Geometry check sheet. Reference: the model listing, model coordinates, mm. Face numbers are marked on the shaded views. A direction names the side the tool comes from. Give positions to 0.01 mm unless a question says otherwise; leave off trailing zeros. Loops run counter-clockwise (first coordinate to the right, second up) from the corner with the lowest first, then second, coordinate; pieces in that order, holes last. Notation, with made-up numbers: (-24.5, 86) -> (0.5, 86) arc R28 ccw to (0.5, 117) -> close; hole circle Ø9 at (52.5, 28). An arc over 180 degrees is marked (long way). One line per item, written item: value. Start each with the question number.
(1) Sectioned sample at C-C, the plane x = 18. Record the cut outline in (y, z), then the cut area to 3 significant figures.
(2) Gauge pin test, flat ends, axial feed: pin 1 Ø2.5 at (x, y) = (20.5, 1) entering from +Z; pin 2 Ø1 at (y, z) = (-1.5, 1) entering from -X; pin 3 Ø1.6 at (y, z) = (2, 43.5) entering from +X. Record the tip position at first contact, or that the pin passes through.
(3) Sectioned sample at B-B, the plane z = 24. Record the cut outline in (x, y).
(4) Tool access check on the marked faces 5 and 6. Record the directions out of +Z, -Z, +X, -X, +Y, -Y that give a thin tool (end or side, any length) a straight path to the whole face; none if there is none.
(5) Draft check along X on the marked faces 1, 2, 3 and 4. Enter one of: pulls with the +X half, pulls with the -X half, needs draft (parallel to the pull), parting line crosses it, or undercut.
(6) Scan lines: line 1 along X through (y, z) = (0, 25); line 2 along X through (y, z) = (1.75, 35.5); line 3 along Y through (x, z) = (40, 22). Record each from-to range of solid material in increasing order. Write a range as from..to.
(7) Sectioned sample at A-A, the plane y = 0. State how many separate pieces and enclosed holes the cut face has, then the cut area to 3 significant figures.
Autodesk Fusion 360 part; units mm, degrees
sketch "Sketch1" plane through (0, 0, 0) normal (0, 0, 1) x (1, 0, 0)
  circle A0 centre (0, 0) radius 2.65
  circle A1 centre (0, 0) radius 5
  line L0 (0, 0) -> (40, 0) construction
  circle A2 centre (40, 0) radius 2.65
  circle A3 centre (40, 0) radius 5
  line L1 (0, -5) -> (40, -5)
  line L2 (0, 5) -> (40, 5)
  dimension "d3" = 5.3
  dimension "d4" = 10
  dimension "d5" = 40
  dimension "d6" = 5.3
  dimension "d7" = 10
extrude "Extrude1" add sketch "Sketch1" along normal blind 45
chamfer "Chamfer1" distance 1 angle 45 2 edges at (-2.4707, 0.9583, 45) (37.5293, 0.9583, 45)
fillet "Fillet1" radius 2.5 2 edges at (-2.4707, 0.9583, 44) (37.5293, 0.9583, 44)
ref_plane "WorkPlane1" through (0, 0, 0) normal (1, 0, 0) x (0, 1, 0)
chamfer "Chamfer2" distance 1 angle 45 2 edges at (-2.4707, 0.9583, 0) (37.5293, 0.9583, 0)
sketch "Sketch2" plane through (0, -5, 0) normal (0, -1, 0) x (1, 0, 0)
  line L0 (0, 0) -> (40, 0)
  line L1 (40, 0) -> (40, 45)
  line L2 (40, 45) -> (0, 45)
  line L3 (0, 45) -> (0, 0)
  line L4 (20, 45) -> (20, 43)
  line L5 (20, 43) -> (16, 43)
  line L6 (16, 43) -> (16, 45)
  line L7 (16, 45) -> (20, 45)
  line L8 (20, 45) -> (20, 43)
  line L9 (20, 45) -> (24, 45)
  line L10 (24, 45) -> (24, 43)
  line L11 (24, 43) -> (20, 43)
  line L12 (20, 43) -> (20, 45)
  line L13 (20, 0) -> (16, 0)
  line L14 (16, 0) -> (16, 2)
  line L15 (16, 2) -> (20, 2)
  line L16 (20, 2) -> (20, 0)
  line L17 (20, 0) -> (24, 0)
  line L18 (24, 0) -> (24, 2)
  line L19 (24, 2) -> (20, 2)
  line L20 (20, 2) -> (20, 0)
  dimension "d15" = 2
  dimension "d16" = 4
  dimension "d17" = 4
  dimension "d18" = 4
  dimension "d19" = 2
  dimension "d20" = 4
  dimension "d21" = 2
extrude "Extrude2" cut sketch "Sketch2" against normal blind 14 contours L0 L13 L14 L15 L16 L20 | L0 L16 L17 L18 L19 L20 | L2 L4 L5 L6 L7 L8 L12 | L2 L4 L8 L9 L10 L11 L12
fillet "Fillet2" radius 2.5 2 edges at (-2.4707, -0.9583, 1) (37.5293, -0.9583, 1)
equation "spacing = 40 mm"
equation "holeSize = 5.30 mm"
equation "d3 = holeSize"
equation "d5 = spacing"
equation "d6 = holeSize"
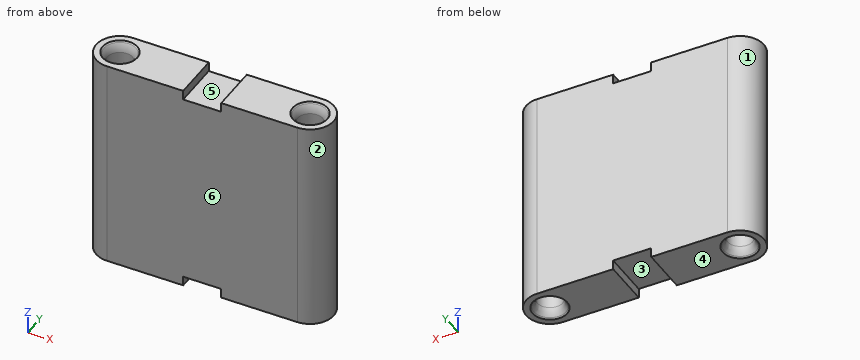
Calculated:
1. outline: (-5, 2) -> (5, 2) -> (5, 43) -> (-5, 43) -> close
1. area: 410 mm2
2. pin 1: stops at z = 43
2. pin 2: stops at x = -4.9
2. pin 3: stops at x = 44.85
3. outline: (0, -5) -> (40, -5) arc R5 ccw to (40, 5) -> (0, 5) arc R5 ccw to start; hole circle Ø5.3 at (0, 0); hole circle Ø5.3 at (40, 0)
4. face 5: +Z, +Y, -Y
4. face 6: +Z, -Z, +X, -X, -Y
5. face 1: pulls with the -X half
5. face 2: pulls with the +X half
5. face 3: undercut
5. face 4: needs draft
6. line 1: x = -5..-2.65, 2.65..37.35, 42.65..45
6. line 2: x = -4.68..-1.99, 1.99..38.01, 41.99..44.68
6. line 3: y = -5..-2.65, 2.65..5
7. separate pieces: 3
7. enclosed holes: 0
7. area: 1,740 mm2
